Geometry: see drawing. Coordinates: mm, zero at the bounding-box minimum. A direction names the side the tool comes from. Round coordinates to 2 decimals unless told otherwise and drop trailing zeros. Write each loop counter-clockwise with the first axis right and the second up, starting at its lowest first coordinate (ties: lowest second). Pieces come first, ordered by that corner, then holes. Notation, with made-up numbers: M 31.25,26.25 L 81.25,26.25 A28 ccw 81.25,51.25 Z; hole C -9,9.5 d6. An arc over 180 degrees is marked long. Use one line per item in the form item = value. Start each with the question number.
Item 1: Reachability of the marked faces 1, 2, 3 and 4 from +Z, -Z, +X, -X, +Y, -Y: full face, straight path, thin tool, end or side. Return the list, or none.
Item 2: Section query C-C (y = 17.5). Return loops of the section in (x, z), and give its area (3 significant figures).
Item 3: Section query B-B (y = 14.85). Return loops of the section in (x, z).
Item 4: Section query D-D (y = 9.85). Return loops of the section in (x, z), and give its area (3 significant figures).
Item 5: Section query A-A (x = 50.5). Return loops of the section in (y, z).
Item 6: Ray query, probe 1 along Y at (x, z) = (50.5, 28.2); probe 2 along Z at (x, y) = (34.5, 3); probe 3 along Y at (x, z) = (3, 28). Return the intervals inside material, ascending.
Item 7: Pin query (flat end, axial travel): pin 1 Ø10 at (x, y) = (28.5, 6) entering from +Z; pin 2 Ø10 at (x, y) = (20, 12) entering from +Z; pin 3 Ø10 at (y, z) = (13, 15.5) entering from +X; pin 4 Ø4.5 at (x, y) = (3.5, 14.85) entering from +Z. Return the tip coordinate at first contact, or that it passes through.
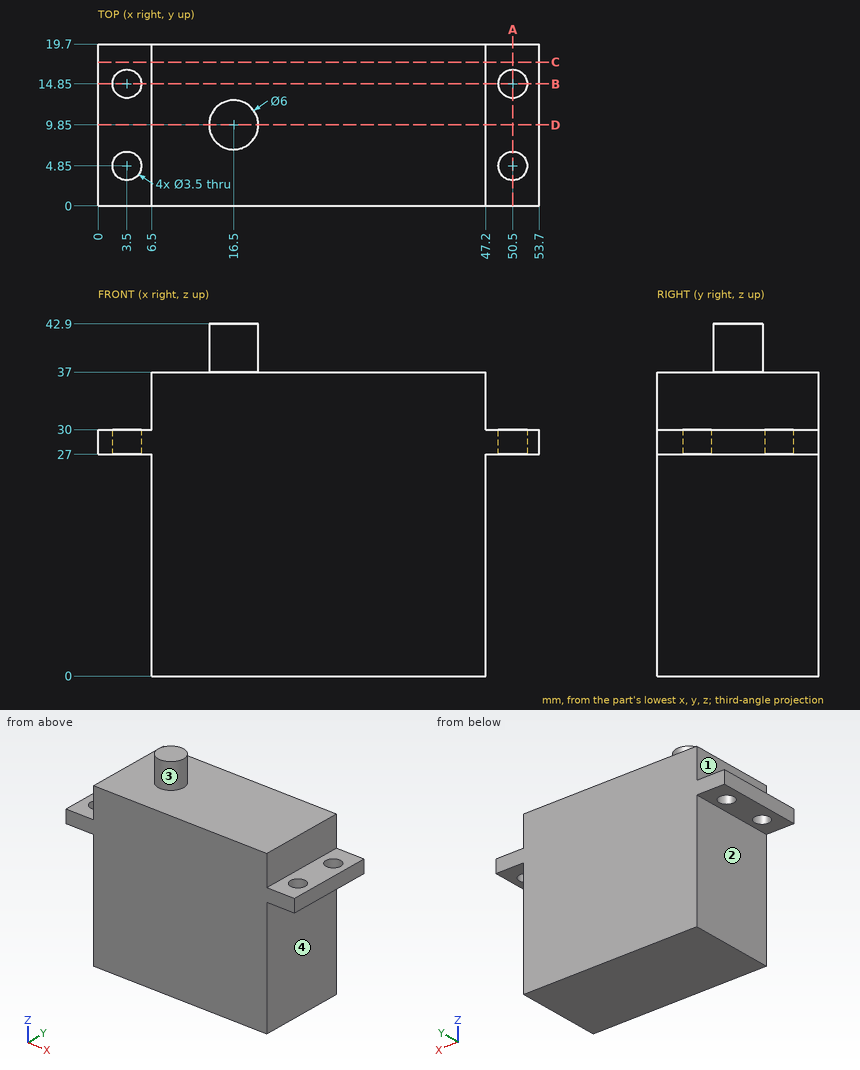
Working result:
q1.face_1 = +Z, -X, +Y, -Y
q1.face_2 = -Z, -X, +Y, -Y
q1.face_3 = +Z
q1.face_4 = -Z, +X, +Y, -Y
q2.outline = M 0,27 L 6.5,27 L 6.5,0 L 47.2,0 L 47.2,27 L 53.7,27 L 53.7,30 L 47.2,30 L 47.2,37 L 6.5,37 L 6.5,30 L 0,30 Z
q2.area = 1,540 mm²
q3.outline = M 0,27 L 1.75,27 L 1.75,30 L 0,30 Z; M 5.25,27 L 6.5,27 L 6.5,0 L 47.2,0 L 47.2,27 L 48.75,27 L 48.75,30 L 47.2,30 L 47.2,37 L 6.5,37 L 6.5,30 L 5.25,30 Z; M 52.25,27 L 53.7,27 L 53.7,30 L 52.25,30 Z
q4.outline = M 0,27 L 6.5,27 L 6.5,0 L 47.2,0 L 47.2,27 L 53.7,27 L 53.7,30 L 47.2,30 L 47.2,37 L 19.5,37 L 19.5,42.9 L 13.5,42.9 L 13.5,37 L 6.5,37 L 6.5,30 L 0,30 Z
q4.area = 1,580 mm²
q5.outline = M 0,27 L 3.1,27 L 3.1,30 L 0,30 Z; M 6.6,27 L 13.1,27 L 13.1,30 L 6.6,30 Z; M 16.6,27 L 19.7,27 L 19.7,30 L 16.6,30 Z
q6.probe_1 = 0 to 3.1, 6.6 to 13.1, 16.6 to 19.7
q6.probe_2 = 0 to 37
q6.probe_3 = 0 to 3.17, 6.53 to 13.17, 16.53 to 19.7
q7.pin_1 = 37
q7.pin_2 = 42.9
q7.pin_3 = 47.2
q7.pin_4 = 30
